from build123d import *

# Parameters (mm, degrees)
BOSS_EXTRUDE1_DEPTH         = 3.175
BOSS_EXTRUDE1_DEPTH_BACK    = 3.175
SKETCH1_R                   = 1.5
SKETCH1_R_2                 = 3
SKETCH2_R                   = 1.75
CUT_EXTRUDE1_DEPTH          = 3
TAP_DRILL_FOR_M3X0_5_TAP1_D = 2.5


with BuildPart() as part:
    # Sketch1 → Boss-Extrude1 (new, two sides: drawn at the far end of the back side and taken through both)
    with BuildSketch(Plane(origin=(0, 0, 0), x_dir=(1, 0, 0), z_dir=(0, 1, 0)).offset(-BOSS_EXTRUDE1_DEPTH_BACK)):
        Polygon((-5, 270), (-5, -15), (5, -15), (5, 270), (12.5, 270), (12.5, 273), (-12.5, 273), (-12.5, 270), align=None)
        with Locations(Location((0, -9.5, 0), (0, 0, 270))):
            Circle(SKETCH1_R, mode=Mode.SUBTRACT)
        with Locations(Location((0, 9.5, 0), (0, 0, 270))):
            Circle(SKETCH1_R, mode=Mode.SUBTRACT)
        with Locations(Location((0, 0, 0), (0, 0, 270))):
            Circle(SKETCH1_R_2, mode=Mode.SUBTRACT)
    extrude(amount=BOSS_EXTRUDE1_DEPTH + BOSS_EXTRUDE1_DEPTH_BACK)

    # Sketch2 → Cut-Extrude1 (cut)
    with BuildSketch(Plane(origin=(0, 0, -273), x_dir=(-1, 0, 0), z_dir=(0, 0, -1))):
        with Locations((-9.5, 0)):
            Circle(SKETCH2_R)
        with Locations(Location((9.5, 0, 0), (0, 0, 180))):
            Circle(SKETCH2_R)
    extrude(amount=-CUT_EXTRUDE1_DEPTH, mode=Mode.SUBTRACT)

    # Tap Drill for M3x0.5 Tap1 (through all)
    with Locations(Plane(origin=(5, 0, 0), x_dir=(0, 0, -1), z_dir=(1, 0, 0))):
        with Locations((0, 0)):
            Hole(TAP_DRILL_FOR_M3X0_5_TAP1_D / 2)


solid = part.part
Geometry check sheet. Reference: the model listing, model coordinates, mm. A direction names the side the tool comes from. Give positions to 0.01 mm unless a question says otherwise; leave off trailing zeros. Order: outer loops, then holes, each group sorted by start corner. A loop starts at its lowest first (then second) coordinate and runs counter-clockwise, first axis right, second up.
1) Cross-section at A-A (y = 0). Record the boundary of the cut face in (x, z).
Results are:
outline: (-12.5, -273) - (-11.25, -273) - (-11.25, -270) - (-12.5, -270) - close; (-7.75, -273) - (7.75, -273) - (7.75, -270) - (5, -270) - (5, -1.25) - (2.73, -1.25) arc R3 cw to (-2.73, -1.25) - (-5, -1.25) - (-5, -270) - (-7.75, -270) - close; (-5, 1.25) - (-2.73, 1.25) arc R3 cw to (2.73, 1.25) - (5, 1.25) - (5, 15) - (-5, 15) - close; (11.25, -273) - (12.5, -273) - (12.5, -270) - (11.25, -270) - close; hole circle Ø3 at (0, -9.5); hole circle Ø3 at (0, 9.5)
2) Material ranges on probe 1 along Z at (x, y) = (-3.7, 0); probe 2 along X at (y, z) = (-1.5, -194.5); probe 3 along X at (y, z) = (1.5, 0), recorded low to high.
Results are:
probe 1: z = -273 to -1.25, 1.25 to 15
probe 2: x = -5 to 5
probe 3: x = -5 to -3, 3 to 5
3) Cross-section at B-B (z = -130.5). Record the boundary of the cut face in (x, y) (3 decimals).
Results are:
outline: (-5, -3.175) - (5, -3.175) - (5, 3.175) - (-5, 3.175) - close
4) Gauge pin test, flat ends, axial feed: pin 1 (3 mm diameter, centred on x = -8, y = -1.5, fed in from +Z); pin 2 (3 mm diameter, centred on x = -9.5, y = 0, fed in from +Z); pin 3 (1 mm diameter, centred on y = 1.5, z = -68, fed in from -X); pin 4 (3 mm diameter, centred on y = 0, z = 0, fed in from +X). Record the tip position at first contact, or that the pin passes through.
Results are:
pin 1: stops at z = -270
pin 2: passes through
pin 3: stops at x = -5
pin 4: stops at x = 5
5) Draft check along Z on faces 4 (the cylindrical face through (0.9, -0.04, 2.86)), 5 (the flat face through (1, 3.175, -130)), 6 (the flat face through (0, 0, 15)). Enter one of: released by +Z, released by -Z, zero draft, split by the parting line, or undercut.
Results are:
face 4: undercut
face 5: zero draft
face 6: released by +Z
6) Tool access check on faces 1 (the flat face through (-7, 0, -270)), 2 (the flat face through (5, 0, -126)), 3 (the flat face through (0, 0, -273)). Record the directions out of +Z, -Z, +X, -X, +Y, -Y that give a thin tool (end or side, any length) a straight path to the whole face; none if there is none.
Results are:
face 1: +Z, -X, +Y, -Y
face 2: +Z, +X, +Y, -Y
face 3: -Z, +X, -X, +Y, -Y
